Can you work these out from the drawing? Everything is in mm from the part's minimum corner. Round coordinates to 2 decimals unless told otherwise and drop trailing zeros. Order: outer loops, then holes, each group sorted by start corner. A loop starts at its lowest first (then second) coordinate and runs counter-clockwise, first axis right, second up. Notation, with made-up numbers: (55.25, -11) -> (80.25, -11) arc R5 ccw to (80.25, -4) -> close; hole circle Ø6 at (-23, 75.5). An arc over 180 degrees is marked (long way). Use a Markdown table: item, result. Add a question column.
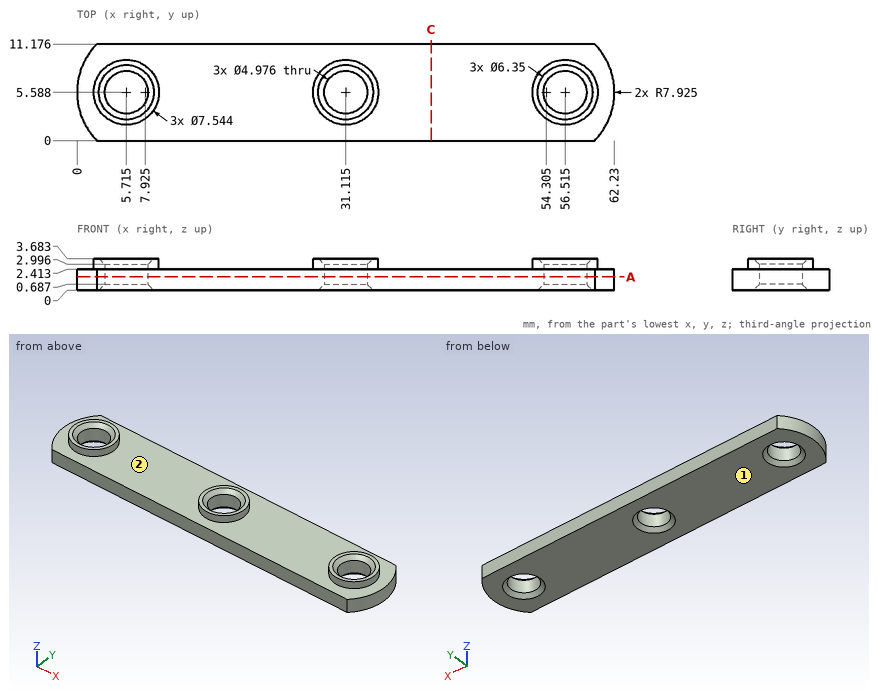
(1) I want a section at C-C on x = 41. List the corners of the cut face in (y, z) for me.
(2) I'm going to push flat-ended pins straight in: P1, Ø3, axis at x = 5.715, y = 5.588, coming from the -Z side; P2, Ø5.5, axis at x = 56.515, y = 5.588, coming from the -Z side (1 decimal); P3, Ø2, axis at x = 15.5, y = 10, coming from the +Z side. Where does each tip first touch, or does it pass through?
(3) Please list where these lines run through material, in increasing order: probe 1 along X at (y, z) = (5, 3.35) (1 decimal); probe 2 along X at (y, z) = (4.25, 0.8); probe 3 along X at (y, z) = (5.5, 3.2) (1 decimal). Write a range as from..to.
(4) If we mould it in two halves opening along X, with no side actions, what happens to the marked faces 1 and 2? For each: pulls with the +X half, pulls with the -X half, needs draft (parallel to the pull), parting line crosses it, or undercut.
(5) I want a section at A-A on z = 1.55. State how many separate pieces and enclosed holes the cut face has, and give its area (3 significant figures).
Output:
| question | item | result |
|---|---|---|
| 1 | outline | (0, 0) -> (11.18, 0) -> (11.18, 2.41) -> (0, 2.41) -> close |
| 2 | P1 | through |
| 2 | P2 | z = 0.4 |
| 2 | P3 | z = 2.41 |
| 3 | probe 1 | 2..2.9, 8.5..9.4, 27.4..28.3, 33.9..34.8, 52.8..53.7, 59.3..60.2 |
| 3 | probe 2 | 0.11..3.62, 7.81..29.02, 33.21..54.42, 58.61..62.12 |
| 3 | probe 3 | 1.9..3, 8.4..9.5, 27.3..28.4, 33.8..34.9, 52.7..53.8, 59.2..60.3 |
| 4 | face 1 | needs draft |
| 4 | face 2 | undercut |
| 5 | separate pieces | 1 |
| 5 | enclosed holes | 3 |
| 5 | area | 621 mm² |
